Can you work these out from the drawing? Everything is in mm from the part's minimum corner. A direction names the side the tool comes from. Give positions to 0.01 mm unless a question says otherwise; leave off trailing zeros. Loops run counter-clockwise (first coordinate to the right, second up) from the corner with the lowest first, then second, coordinate; pieces in that order, holes last. Notation, with made-up numbers: M -8,-15.5 L 43,-15.5 A35 ccw 43,20.5 Z; hole C 20,9 d11. An arc over 180 degrees is marked long. Use CSV: the item, a comma, the result in double quotes.
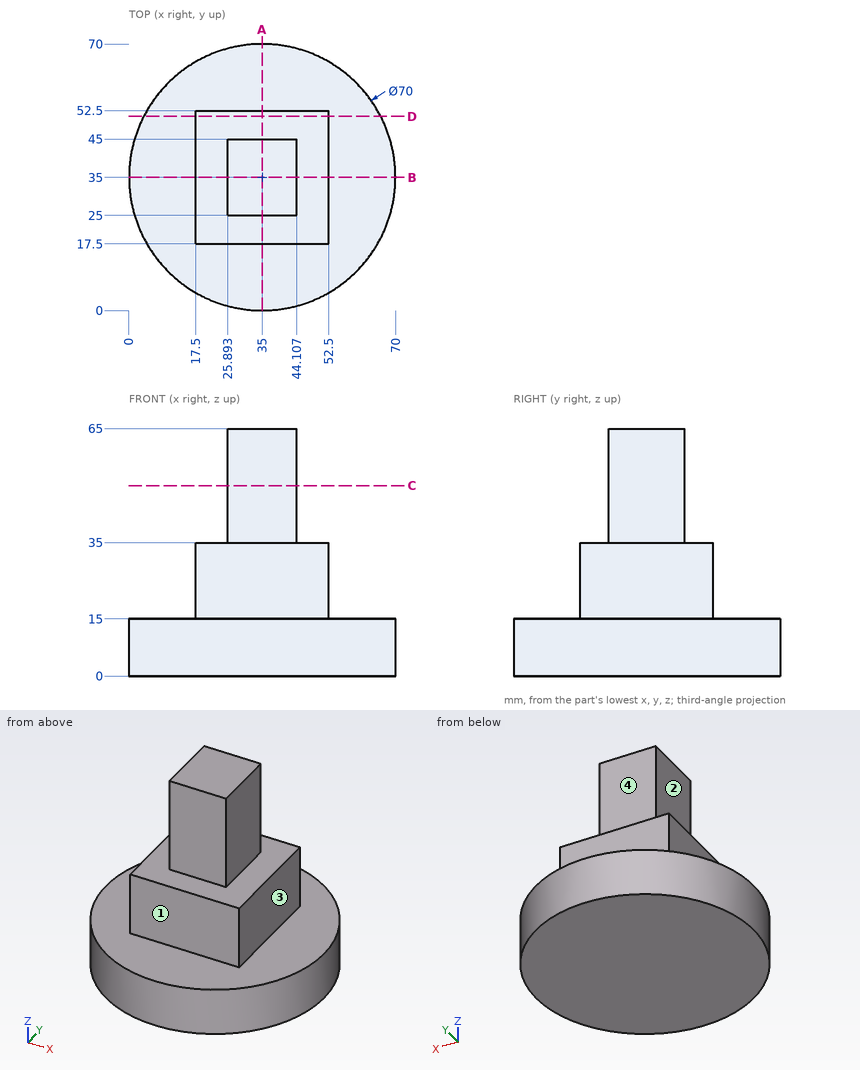
Q1. I want a section at D-D, the plane y = 51. Please give me the cut outline in (x, z), then the cut area to 3 significant figures.
Model answer:
outline,"M 3.87,0 L 66.13,0 L 66.13,15 L 52.5,15 L 52.5,35 L 17.5,35 L 17.5,15 L 3.87,15 Z"
area,"1,630 mm2"
Q2. I want a section at C-C, the plane z = 50. Please give me the cut outline in (x, y), then the cut area to 3 significant figures.
Model answer:
outline,"M 25.89,25 L 44.11,25 L 44.11,45 L 25.89,45 Z"
area,"364 mm2"
Q3. For the marked faces 1, 2, 3 and 4, which set-ups out of +Z, -Z, +X, -X, +Y, -Y let a thin tool reach every point of the face, with its end or its side?
Model answer:
face 1,"+Z, +X, -X, -Y"
face 2,"+Z, -X, +Y, -Y"
face 3,"+Z, +X, +Y, -Y"
face 4,"+Z, +X, -X, +Y"
Q4. I'm going to push flat-ended pins straight in: P1, Ø8, axis at x = 42.5, z = 20.5, coming from the -Y side; P2, Ø5.5, axis at x = 37, z = 48.5, coming from the -Y side; P3, Ø5.5, axis at x = 35.5, z = 45.5, coming from the +Y side. Where does each tip first touch, or does it pass through?
Model answer:
P1,"y = 17.5"
P2,"y = 25"
P3,"y = 45"
Q5. Please list where these lines run through material, in increasing order: L1, parallel to Z at x = 49.5, y = 19; L2, parallel to Y at x = 41.5, z = 44; L3, parallel to Z at x = 59, y = 40. Write a range as from..to.
Model answer:
L1,"0..35"
L2,"25..45"
L3,"0..15"
Q6. I want a section at B-B, the plane y = 35. Please give me the cut outline in (x, z).
Model answer:
outline,"M 0,0 L 70,0 L 70,15 L 52.5,15 L 52.5,35 L 44.11,35 L 44.11,65 L 25.89,65 L 25.89,35 L 17.5,35 L 17.5,15 L 0,15 Z"
Q7. I want a section at A-A, the plane x = 35. Please give me the cut outline in (y, z), then the cut area to 3 significant figures.
Model answer:
outline,"M 0,0 L 70,0 L 70,15 L 52.5,15 L 52.5,35 L 45,35 L 45,65 L 25,65 L 25,35 L 17.5,35 L 17.5,15 L 0,15 Z"
area,"2,350 mm2"
